```python
from build123d import *

# Parameters (mm, degrees)
F1_DEPTH    = 10
F2_C1_SIZE2 = 5
F2_C1_SIZE  = 3
F2_C2_SIZE2 = 5
F2_C2_SIZE  = 3
F2_C3_SIZE2 = 5
F2_C3_SIZE  = 3
F3_T1_DEPTH = 12.1433659759
F5_SIZE     = 1
F7_DEPTH    = 10.001


# Not quite as in the source:
# - a fillet or chamfer that OpenCascade refuses, or shapes differently, is made with other operations: its cross-section is extruded or revolved along the edge and cut away or added
# - two fillets or chamfers of one size are made in one step


with BuildPart() as f1:
    # F0 (on Top) → F1 (new body)
    with BuildSketch(Plane.XY):
        Polygon((50, 40), (0, 40), (0, 0), (40, 0), (50, 10), align=None)
    extrude(amount=F1_DEPTH)

    # F2: chamfer of 5 x 3 on 3 edges, made by hand

    # F2_c1
    f2_c1_edges = [f1.edges().sort_by_distance(p)[0] for p in [
        (25, 40, 10),
    ]]
    f2_c1_side = f1.faces().sort_by_distance((25, 40, 9.94))[0]
    chamfer(f2_c1_edges, length=F2_C1_SIZE, length2=F2_C1_SIZE2, reference=f2_c1_side)

    # F2_c2
    f2_c2_edges = [f1.edges().sort_by_distance(p)[0] for p in [
        (0, 17.5, 10),
    ]]
    f2_c2_side = f1.faces().sort_by_distance((0, 17.5, 9.94))[0]
    chamfer(f2_c2_edges, length=F2_C2_SIZE, length2=F2_C2_SIZE2, reference=f2_c2_side)

    # F2_c3
    f2_c3_edges = [f1.edges().sort_by_distance(p)[0] for p in [
        (45, 5, 10),
    ]]
    f2_c3_side = f1.faces().sort_by_distance((44.9575735931, 5.0424264069, 10))[0]
    chamfer(f2_c3_edges, length=F2_C3_SIZE, length2=F2_C3_SIZE2, reference=f2_c3_side)

    # F3: chamfer of 1 on 1 edges, made by hand

    # F3_s2 → F3_t1 (cut)
    with BuildSketch(Plane.XY.offset(-2.571682988)):
        Polygon((1, 40), (0, 39), (0, 40), align=None)
    extrude(amount=F3_T1_DEPTH, mode=Mode.SUBTRACT)

    # F5
    f5_edges = [f1.edges().sort_by_distance(p)[0] for p in [
        (50, 25, 0),
        (45, 5, 0),
        (20, 0, 0),
        (0, 19.5, 0),
        (0.5, 39.5, 0),
        (25.5, 40, 0),
    ]]
    chamfer(f5_edges, length=F5_SIZE)

    # F6 (on face) → F7 (cut, through all)
    with BuildSketch(Plane.XY.offset(10)):
        Polygon((9, 31), (9, 4), (34.1005050634, 4), (45.3436888701, 15.2431838067), (45.3436888701, 31), align=None)
    extrude(amount=-F7_DEPTH, mode=Mode.SUBTRACT)


solid = f1.part
```
Could you check a few things on this model? Use its own coordinates, in mm. A direction names the side the tool comes from. Coordinates: 2 decimals unless noted, no trailing zeros. Order: outer loops, then holes, each group sorted by start corner. A loop starts at its lowest first (then second) coordinate and runs counter-clockwise, first axis right, second up. Notation, with made-up numbers: M 8.5,64.5 L 49.5,64.5 A12 ccw 49.5,84.5 Z; hole C 41.25,-2 d7. An arc over 180 degrees is marked long. Use a Markdown table: item, result. Add a question column.
Q1. We'd pull the mould along X, two halves only. Please class faces 3 (the flat face through (9, 18, 5)), 4 (the flat face through (50, 25, 5)), 5 (the flat face through (26, 40, 4)): pulls with the +X half, pulls with the -X half, needs draft (parallel to the pull), parting line crosses it, or undercut.
Q2. I want a section at B-B on x = 29. List the corners of the cut face in (y, z) for me, then the cut area to 4 significant figures.
Q3. I want a section at A-A on y = 24. List the corners of the cut face in (x, z) for me.
Q4. I want a section at C-C on z = 2. List the corners of the cut face in (x, y) for me, then the cut area to 3 significant figures.
Q5. I'm going to push a flat-ended pin straight in: pin 1 (4 mm diameter, centred on x = 43, z = 8, fed in from -Y). Where does the tip first touch, or does it pass through?
Q6. I want a section at D-D on y = 32. List the corners of the cut face in (x, z) for me.
Q7. Which directions (+Z, -Z, +X, -X, +Y, -Y) give clear straight access to the entire face, cutting with the end or side of a thin tool? Please do faces 1 (the flat face through (2.5, 20, 8.5)), 2 (the flat face through (39.6, 9.5, 5.1)).
Q8. If I drill on L1, parallel to Y at x = 27, z = 6; L2, parallel to X at y = 21, z = 6.5; L3, parallel to X at y = 14.5, z = 3.5, over which ranges is the centre line in solid material (lowest first)?
Checked values:
| question | item | result |
|---|---|---|
| 1 | face 3 | undercut |
| 1 | face 4 | pulls with the +X half |
| 1 | face 5 | needs draft |
| 2 | outline | M 0,1 L 1,0 L 4,0 L 4,10 L 0,10 Z; M 31,0 L 39,0 L 40,1 L 40,7 L 35,10 L 31,10 Z |
| 2 | area | 121.5 mm² |
| 3 | outline | M 0,1 L 1,0 L 9,0 L 9,10 L 5,10 L 0,7 Z; M 45.34,0 L 49,0 L 50,1 L 50,10 L 45.34,10 Z |
| 4 | outline | M 0,0 L 40,0 L 50,10 L 50,40 L 1,40 L 0,39 Z; hole M 9,4 L 34.1,4 L 45.34,15.24 L 45.34,31 L 9,31 Z |
| 4 | area | 1,030 mm² |
| 5 | pin 1 | y = 2.92 |
| 6 | outline | M 0,1 L 1,0 L 49,0 L 50,1 L 50,10 L 5,10 L 0,7 Z |
| 7 | face 1 | +Z, -X, +Y, -Y |
| 7 | face 2 | +Z, -Z |
| 8 | L1 | 0 to 4, 31 to 40 |
| 8 | L2 | 0 to 9, 45.34 to 50 |
| 8 | L3 | 0 to 9, 44.6 to 50 |
